The model under review builds one solid part; all positions refer to its coordinate system, in mm. Round coordinates to 2 decimals unless told otherwise and drop trailing zeros. Order: outer loops, then holes, each group sorted by start corner. A loop starts at its lowest first (then second) coordinate and runs counter-clockwise, first axis right, second up. Notation, with made-up numbers: M 65.5,-11.75 L 105.5,-11.75 A12 cw 105.5,-7.75 Z; hole C 71,20.5 d3. An arc over 180 degrees is marked long. Answer as a JSON object with one key per item and string values. Group by question number.
1. Add section A-A on z = -18. State the section outline as (x, y) points.
2. Clearance check with flat-ended pins moving along their axes: P1, Ø2.5, axis at x = 1, y = 33.5, coming from the -Z side; P2, Ø2, axis at x = -2, y = 9, coming from the +Z side; P3, Ø1.6, axis at x = 0, z = -59.5, coming from the +Y side. State where each tip first meets the part, or that it passes through.
3. Add section D-D on y = 28.5. State the section outline as (x, z) points (3 decimals).
4. To check wall thickness, follow probe 1 along Y at (x, z) = (-0.6, 0) (3 decimals); probe 2 along Z at (x, y) = (-2.5, 20) (1 decimal); probe 3 along Z at (x, y) = (1.5, 18.5) (3 decimals). State the ranges of each line that lie inside material, in increasing order. Write a range as [from, to].
5. Add section B-B on y = 19.5. State the section outline as (x, z) points (1 decimal).
6. Add section C-C on z = -26. State the section outline as (x, y) points, and give its area (3 significant figures).
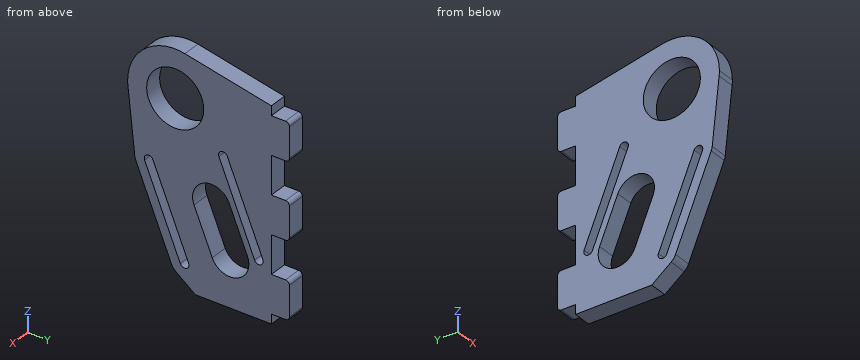
```python
from build123d import *

# Parameters (mm, degrees)
SKETCH1_R              = 9.525
BOSS_EXTRUDE1_DEPTH    = 3
CUT_EXTRUDE1_DEPTH     = 69.596761039
SKETCH3_W              = 6
SKETCH3_H              = 12.7
BOSS_EXTRUDE2_DEPTH    = 6
FILLET1_R              = 1.27
LPATTERN1_COUNT        = 3
LPATTERN1_PITCH        = 25.4
FILLET1_OF_LPATTERN1_R = 1.27


with BuildPart() as part:
    # Sketch1 → Boss-Extrude1 (new, symmetric)
    with BuildSketch(Plane(origin=(0, 0, 0), x_dir=(0, 0, -1), z_dir=(1, 0, 0))):
        with BuildLine():
            Line((-15.540953853, 3.23950279), (-9.525, 32.1))
            Line((-9.525, 32.1), (60.325, 32.1))
            Line((60.325, 32.1), (60.325, -15.875))
            Line((60.325, -15.875), (0, -15.875))
            ThreePointArc((0, -15.875), (-12.317522717, -10.014702148), (-15.540953853, 3.23950279))
        make_face()
        Circle(SKETCH1_R, mode=Mode.SUBTRACT)
    extrude(amount=BOSS_EXTRUDE1_DEPTH, both=True)

    # Sketch2 → Cut-Extrude1 (cut, through all)
    with BuildSketch(Plane(origin=(3, 0, 0), x_dir=(0, 0, -1), z_dir=(1, 0, 0))):
        with BuildLine():
            Line((1.676231888, -15.786255783), (23.396510982, -13.47993154))
            ThreePointArc((23.396510982, -13.47993154), (24.056064004, -13.361605673), (24.691925535, -13.150202478))
            Line((24.691925535, -13.150202478), (53.43843719, -1.24300748))
            ThreePointArc((53.43843719, -1.24300748), (54.494953994, -0.633102763), (55.357708418, 0.229374093))
            Line((55.357708418, 0.229374093), (60.325, 6.7))
            Line((60.325, 6.7), (60.325, -15.875))
            Line((60.325, -15.875), (0, -15.875))
            ThreePointArc((0, -15.875), (0.839289711, -15.852798421), (1.676231888, -15.786255783))
        make_face()
        with BuildLine():
            Line((26.903135362, 18.016834009), (41.56972294, 24.091933498))
            ThreePointArc((41.56972294, 24.091933498), (49.866397767, 20.655338262), (46.429802531, 12.358663435))
            Line((46.429802531, 12.358663435), (31.763214953, 6.283563946))
            ThreePointArc((31.763214953, 6.283563946), (23.466540126, 9.720159182), (26.903135362, 18.016834009))
        make_face()
        with BuildLine():
            Line((22.328855341, -7.445246365), (51.075366995, 4.461948633))
            ThreePointArc((51.075366995, 4.461948633), (53.035211442, 3.650154483), (52.223417292, 1.690310036))
            Line((52.223417292, 1.690310036), (23.476905638, -10.216884962))
            ThreePointArc((23.476905638, -10.216884962), (21.51706119, -9.405090812), (22.328855341, -7.445246365))
        make_face()
        with BuildLine():
            Line((12.055034553, 17.357951117), (40.801546208, 29.265146115))
            ThreePointArc((40.801546208, 29.265146115), (42.761390655, 28.453351965), (41.949596505, 26.493507518))
            Line((41.949596505, 26.493507518), (13.203084851, 14.58631252))
            ThreePointArc((13.203084851, 14.58631252), (11.243240403, 15.39810667), (12.055034553, 17.357951117))
        make_face()
    extrude(amount=-CUT_EXTRUDE1_DEPTH, mode=Mode.SUBTRACT)

    # Sketch3 → Boss-Extrude2 (add)
    with BuildSketch(Plane(origin=(0, 32.1, 0), x_dir=(1, 0, 0), z_dir=(0, 1, 0))):
        Rectangle(SKETCH3_W, SKETCH3_H)
    boss_extrude2 = extrude(amount=BOSS_EXTRUDE2_DEPTH)

    # Fillet1
    fillet1_edges = [part.edges().sort_by_distance(p)[0] for p in [
        (0, 38.1, -6.35),
        (0, 38.1, 6.35),
    ]]
    fillet(fillet1_edges, radius=FILLET1_R)

    # LPattern1: Boss-Extrude2 ×3
    with Locations(*[(0, 0, -i * LPATTERN1_PITCH) for i in range(1, LPATTERN1_COUNT)]):
        add(boss_extrude2)

    # Fillet1 of LPattern1
    fillet1_of_lpattern1_edges = [part.edges().sort_by_distance(p)[0] for p in [
        (0, 38.1, -31.75),
        (0, 38.1, -19.05),
        (0, 38.1, -57.15),
        (0, 38.1, -44.45),
    ]]
    fillet(fillet1_of_lpattern1_edges, radius=FILLET1_OF_LPATTERN1_R)


solid = part.part
```
Recorded:
{
 "1": {"outline": "M -3,-14.05 L 3,-14.05 L 3,16.57 L -3,16.57 Z; M -3,19.82 L 3,19.82 L 3,32.1 L -3,32.1 Z"},
 "2": {"P1": "stops at z = -57.15", "P2": "stops at z = 14.55", "P3": "stops at y = 32.1"},
 "3": {"outline": "M -3,-60.325 L 3,-60.325 L 3,-42.741 L -3,-42.741 Z; M -3,-38.954 L 3,-38.954 L 3,10.275 L -3,10.275 Z"},
 "4": {"probe 1": "y = [-15.875, -9.525], [9.525, 38.1]", "probe 2": "z = [-60.3, -50.1], [-31.7, -26.3], [-18.4, 12]", "probe 3": "z = [-60.325, -50.344], [-28.07, -22.652], [-14.812, 12.36]"},
 "5": {"outline": "M -3,-60.3 L 3,-60.3 L 3,-50.2 L -3,-50.2 Z; M -3,-30.5 L 3,-30.5 L 3,-25.1 L -3,-25.1 Z; M -3,-17.2 L 3,-17.2 L 3,12.2 L -3,12.2 Z"},
 "6": {"outline": "M -3,-12.61 L 3,-12.61 L 3,-9.17 L -3,-9.17 Z; M -3,-5.92 L 3,-5.92 L 3,6.75 L -3,6.75 Z; M -3,17.56 L 3,17.56 L 3,19.89 L -3,19.89 Z; M -3,23.13 L 3,23.13 L 3,38.1 L -3,38.1 Z", "area": "200 mm²"}
}
